Autodesk Inventor part; units mm, degrees
ref_plane "YZ Plane" through (0, 0, 0) normal (1, 0, 0) x (0, 1, 0)
ref_plane "XZ Plane" through (0, 0, 0) normal (0, 1, 0) x (-1, 0, 0)
ref_plane "XY Plane" through (0, 0, 0) normal (0, 0, 1) x (1, 0, 0)
sketch "Sketch1" plane through (0, 0, 0) normal (0, 1, 0) x (-1, 0, 0)
  line L0 (14.25, 24) -> (-14.25, 24)
  line L1 (-14.25, 24) -> (-14.25, -24)
  line L2 (-14.25, -24) -> (14.25, -24)
  line L3 (14.25, -24) -> (14.25, 24)
  line L4 (14.25, 24) -> (-14.25, -24) construction
  line L5 (-14.25, 24) -> (14.25, -24) construction
  point P0 (0, 0)
  dimension "d0" = 28.5
  dimension "d1" = 48
extrude "Extrusion1" add sketch "Sketch1" along normal blind 4
sketch "Sketch2" plane through (0, 4, 0) normal (0, 1, 0) x (1, 0, 0)
  circle A0 centre (0, -13) radius 8.25
  circle A1 centre (0, 13) radius 8.25
  line L0 (14.25, 24) -> (-14.25, 24)
  line L1 (-14.25, 24) -> (-14.25, -24)
  point P0 (0, 0)
  dimension "d4" = 16.5
  dimension "d5" = 16.5
  dimension "d6" = 26
  dimension "d7" = 11
  dimension "d8" = 14.25
  dimension "d9" = 14.25
extrude "Extrusion2" cut sketch "Sketch2" against normal blind 4
sketch "Sketch3" plane through (0, 4, 0) normal (0, 1, 0) x (1, 0, 0)
  line L0 (14.25, -24) -> (10.25, -24)
  line L1 (10.25, -24) -> (10.25, 24)
  line L2 (10.25, 24) -> (14.25, 24)
  line L3 (14.25, 24) -> (14.25, -24)
  line L4 (14.25, -24) -> (10.25, 24) construction
  line L5 (10.25, -24) -> (14.25, 24) construction
  line L6 (14.25, -24) -> (14.25, 24)
  line L7 (14.25, 24) -> (-14.25, 24)
  point P0 (0, 0)
  point P1 (12.25, 0)
  dimension "d12" = 48
  dimension "d13" = 4
extrude "Extrusion3" add sketch "Sketch3" along normal blind 17
sketch "Sketch4" plane through (0, 4, 0) normal (0, 1, 0) x (1, 0, 0)
  line L0 (-14.25, -24) -> (-10.25, -24)
  line L1 (-10.25, -24) -> (-10.25, -11)
  line L2 (-10.25, -11) -> (-14.25, -11)
  line L3 (-14.25, -11) -> (-14.25, -24)
  line L4 (-14.25, -24) -> (10.25, -24)
  line L5 (-14.25, 24) -> (-14.25, -24)
  line L6 (-14.25, 24) -> (-10.25, 24)
  line L7 (-10.25, 24) -> (-10.25, 11)
  line L8 (-10.25, 11) -> (-14.25, 11)
  line L9 (-14.25, 11) -> (-14.25, 24)
  point P0 (0, 0)
  dimension "d16" = 4
  dimension "d17" = 13
  dimension "d18" = 4
  dimension "d19" = 13
extrude "Extrusion4" add sketch "Sketch4" along normal blind 15
sketch "Sketch5" plane through (-14.25, 0, -24) normal (-1, 0, 0) x (0, 0, 1)
  line L0 (41.5, 15.5) -> (48, 15.5)
  line L1 (48, 15.5) -> (48, 11)
  line L2 (48, 11) -> (41.5, 11)
  line L3 (41.5, 11) -> (41.5, 15.5)
  line L4 (35, 4) -> (35, 19)
  line L5 (0, 0) -> (48, 0)
  line L6 (0, 15.5) -> (6.5, 15.5)
  line L7 (6.5, 15.5) -> (6.5, 11)
  line L8 (6.5, 11) -> (0, 11)
  line L9 (0, 11) -> (0, 15.5)
  line L10 (13, 4) -> (13, 19)
  line L11 (48, 0) -> (48, 19)
  line L12 (0, 0) -> (0, 19)
  point P0 (24, 0)
  dimension "d22" = 6.5
  dimension "d23" = 4.5
  dimension "d24" = 11
  dimension "d25" = 6.5
  dimension "d26" = 4.5
  dimension "d27" = 11
extrude "Extrusion5" cut sketch "Sketch5" against normal blind 4
sketch "Sketch6" plane through (10.25, 4, -24) normal (-1, 0, 0) x (0, 0, 1)
  point P0 (24, -4)
sketch "Sketch7" plane through (10.25, 4, -24) normal (-1, 0, 0) x (0, 0, 1)
  circle A0 centre (24, 8.5) radius 2.625
  line L0 (13, 0) -> (35, 0)
  point P0 (24, -4)
  dimension "d30" = 5.25
  dimension "d31" = 8.5
extrude "Extrusion6" cut sketch "Sketch7" against normal blind 2
sketch "Sketch8" plane through (12.25, 12.5, 0) normal (-1, 0, 0) x (0, 0, 1)
  circle A0 centre (0, 0) radius 2.625
  circle A1 centre (0, 0) radius 1
  point P0 (0, -12.5)
  dimension "d34" = 2
extrude "Extrusion7" cut sketch "Sketch8" against normal blind 2 contours A1
sketch "Sketch9" plane through (0, 4, 0) normal (0, 1, 0) x (1, 0, 0)
  line L0 (-10.25, -24) -> (10.25, -24)
  line L1 (10.25, -24) -> (10.25, -22.5)
  line L2 (10.25, -22.5) -> (-10.25, -22.5)
  line L3 (-10.25, -22.5) -> (-10.25, -24)
  line L4 (-10.25, -11) -> (-10.25, -24)
  line L5 (-10.25, -24) -> (10.25, -24)
  line L6 (-10.25, 22.5) -> (10.25, 22.5)
  line L7 (10.25, 22.5) -> (10.25, 24)
  line L8 (10.25, 24) -> (-10.25, 24)
  line L9 (-10.25, 24) -> (-10.25, 22.5)
  line L10 (-10.25, 24) -> (-10.25, 11)
  line L11 (10.25, 24) -> (-10.25, 24)
  point P0 (0, 0)
  dimension "d37" = 20.5
  dimension "d38" = 1.5
  dimension "d39" = 1.5
  dimension "d40" = 20.5
extrude "Extrusion8" add sketch "Sketch9" along normal blind 3.5
sketch "Sketch10" plane through (14.25, 0, 24) normal (1, 0, 0) x (0, 0, -1)
  line L0 (48, 15.5) -> (41.5, 15.5)
  line L1 (41.5, 15.5) -> (41.5, 11)
  line L2 (41.5, 11) -> (48, 11)
  line L3 (48, 11) -> (48, 15.5)
  line L4 (41.5, 11) -> (41.5, 15.5)
  line L5 (41.5, 15.5) -> (48, 15.5)
  line L6 (48, 0) -> (48, 21)
  line L7 (0, 0) -> (48, 0)
  point P0 (24, 0)
  dimension "d43" = 4.5
  dimension "d44" = 6.5
  dimension "d45" = 11
sketch "Sketch11" plane through (14.25, 0, 24) normal (1, 0, 0) x (0, 0, -1)
  line L0 (6.5, 15.5) -> (0, 15.5)
  line L1 (0, 15.5) -> (0, 11)
  line L2 (0, 11) -> (6.5, 11)
  line L3 (6.5, 11) -> (6.5, 15.5)
  line L4 (0, 0) -> (48, 0)
  line L5 (0, 0) -> (0, 21)
  point P0 (24, 0)
  dimension "d46" = 6.5
  dimension "d47" = 4.5
  dimension "d48" = 11
extrude "Extrusion9" cut sketch "Sketch10" against normal blind 4
extrude "Extrusion10" cut sketch "Sketch11" against normal blind 4
properties part number "Ultrasound Mount 4"
Input: part model. Units: mm. Frame: model coordinates. A direction names the side the tool comes from. Round coordinates to 2 decimals unless told otherwise and drop trailing zeros. Order: outer loops, then holes, each group sorted by start corner. A loop starts at its lowest first (then second) coordinate and runs counter-clockwise, first axis right, second up.
1. Material intervals for line 1 (Z direction, x = 0, y = 2.05); line 2 (X direction, y = 4.25, z = 21.5); line 3 (X direction, y = 3.05, z = 13), sorted ascending.
The answers:
line 1: z = -24 to -21.25, -4.75 to 4.75, 21.25 to 24
line 2: x = -14.25 to -10.25, 10.25 to 14.25
line 3: x = -14.25 to -8.25, 8.25 to 14.25
2. Cut plane A-A, the plane y = 12.5. Output: boundary loops of the cut face in (x, z) (3 decimals).
The answers:
outline: (-14.25, -17.5) - (-10.25, -17.5) - (-10.25, -11) - (-14.25, -11) - close; (-14.25, 11) - (-10.25, 11) - (-10.25, 17.5) - (-14.25, 17.5) - close; (10.25, -17.5) - (14.25, -17.5) - (14.25, -1) - (12.25, -1) - (12.25, -2.625) - (10.25, -2.625) - close; (10.25, 2.625) - (12.25, 2.625) - (12.25, 1) - (14.25, 1) - (14.25, 17.5) - (10.25, 17.5) - close
3. Set-up query: faces 5 (the face through (12, 15.5, 21)), 6 (the face through (-10.25, 11, 16)), 7 (the face through (-12, 13, -17.5)). Return all of +Z, -Z, +X, -X, +Y, -Y with unobstructed straight access to the full face (end or side cutting, diameter ignored); none if empty.
The answers:
face 5: +Z, +X, -X
face 6: +Y
face 7: -Z, +X, -X
4. Pin query (flat end, axial travel): P1, Ø4, axis at y = 6.5, z = -8.5, coming from the -X side; P2, Ø1.2, axis at x = -13, z = -17.5, coming from the +Y side; P3, Ø2, axis at x = -12.5, y = 14, coming from the +Z side. Return the tip coordinate at first contact, or that it passes through.
The answers:
P1: stops at x = 10.25
P2: stops at y = 19
P3: stops at z = 17.5
5. Cut plane C-C, the plane y = 18.25. Output: boundary loops of the cut face in (x, z).
The answers:
outline: (-14.25, -24) - (-10.25, -24) - (-10.25, -11) - (-14.25, -11) - close; (-14.25, 11) - (-10.25, 11) - (-10.25, 24) - (-14.25, 24) - close; (10.25, -24) - (14.25, -24) - (14.25, 24) - (10.25, 24) - close
6. Mould query, pull axis Y, two halves, no side actions, for faces 1 (the face through (-12, 11, -21)), 2 (the face through (12, 15.5, -21)), 3 (the face through (0, 6, 22.5)), 4 (the face through (0, 0, 0)). Classes: released by +Y, released by -Y, zero draft, split by the parting line, or undercut.
The answers:
face 1: undercut
face 2: undercut
face 3: zero draft
face 4: released by -Y
7. Cut plane B-B, the plane z = 13. Output: boundary loops of the cut face in (x, y).
The answers:
outline: (-14.25, 0) - (-8.25, 0) - (-8.25, 4) - (-10.25, 4) - (-10.25, 19) - (-14.25, 19) - close; (8.25, 0) - (14.25, 0) - (14.25, 21) - (10.25, 21) - (10.25, 4) - (8.25, 4) - close
8. Cut plane D-D, the plane x = 9.75. Output: boundary loops of the cut face in (y, z), then the cut area to 4 significant figures.
The answers:
outline: (0, -24) - (7.5, -24) - (7.5, -22.5) - (4, -22.5) - (4, 22.5) - (7.5, 22.5) - (7.5, 24) - (0, 24) - close
area: 202.5 mm2
